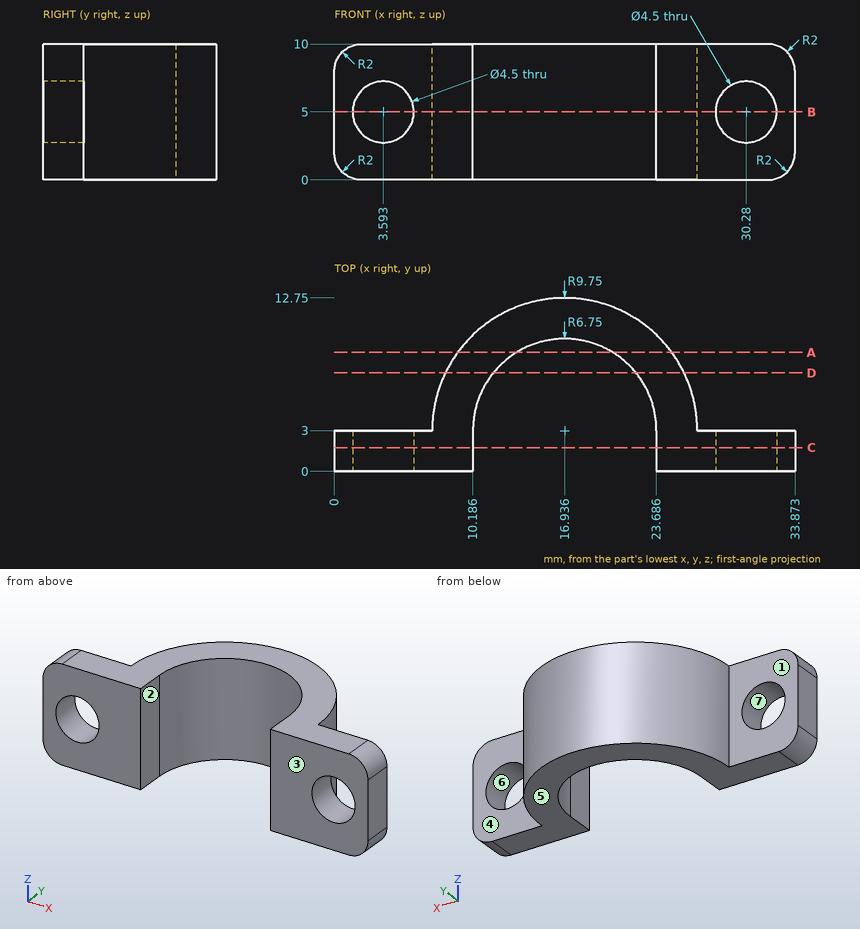
Part print with two shaded views. Sizes in mm from the minimum x, y, z corner. A direction names the side the tool comes from. Give positions to 0.01 mm unless a question says otherwise; leave off trailing zeros. Order: outer loops, then holes, each group sorted by start corner. A loop starts at its lowest first (then second) coordinate and runs counter-clockwise, first axis right, second up.
1) Pin check, flat tips, straight feed: pin 1 (1 mm diameter, centred on x = 22, z = 9, fed in from -Y); pin 2 (3.5 mm diameter, centred on x = 31.5, z = 6, fed in from +Y). Stop position of each tip, or through.
2) Saw through at B-B, the plane z = 5. Write the cut outline in (x, y).
3) Wall check: probe 1 along X at (y, z) = (2.2, 5); probe 2 along Y at (x, z) = (6.5, 9.5); probe 3 along X at (y, z) = (7.75, 6.5). Give the ranges that are in metal, low to high.
4) Saw through at A-A, the plane y = 8.75. Write the cut outline in (x, z).
5) Saw through at D-D, the plane y = 7.25. Write the cut outline in (x, z).
6) Saw through at C-C, the plane y = 1.75. Write the cut outline in (x, z).
7) Mould opens along Z. For the marked faces 4, 5, 6 and 7 say: +Z half, -Z half, draft (parallel to the pull), parting line (faces both ways), or undercut.
8) 3-axis set-ups, long thin cutter, end or side, ignore diameter. For the marked faces 1, 2 and 3: which of +Z, -Z, +X, -X, +Y, -Y reach the whole face in a straight line?
Computed:
1. pin 1: stops at y = 6.82
1. pin 2: stops at y = 3
2. outline: (0, 0) - (1.34, 0) - (1.34, 3) - (0, 3) - close; (5.84, 0) - (10.19, 0) - (10.19, 3) arc R6.75 cw to (23.69, 3) - (23.69, 0) - (28.03, 0) - (28.03, 3) - (26.69, 3) arc R9.75 ccw to (7.19, 3) - (5.84, 3) - close; (32.53, 0) - (33.87, 0) - (33.87, 3) - (32.53, 3) - close
3. probe 1: x = 0 to 1.34, 5.84 to 10.19, 23.69 to 28.03, 32.53 to 33.87
3. probe 2: y = 0 to 3
3. probe 3: x = 8.42 to 12.14, 21.73 to 25.45
4. outline: (9.06, 0) - (13.4, 0) - (13.4, 10) - (9.06, 10) - close; (20.47, 0) - (24.81, 0) - (24.81, 10) - (20.47, 10) - close
5. outline: (8.16, 0) - (11.69, 0) - (11.69, 10) - (8.16, 10) - close; (22.18, 0) - (25.71, 0) - (25.71, 10) - (22.18, 10) - close
6. outline: (0, 2) arc R2 ccw to (2, 0) - (10.19, 0) - (10.19, 10) - (2, 10) arc R2 ccw to (0, 8) - close; (23.69, 0) - (31.87, 0) arc R2 ccw to (33.87, 2) - (33.87, 8) arc R2 ccw to (31.87, 10) - (23.69, 10) - close; hole circle Ø4.5 at (3.59, 5); hole circle Ø4.5 at (30.28, 5)
7. face 4: draft
7. face 5: -Z half
7. face 6: undercut
7. face 7: undercut
8. face 1: +Z, -Z, -X, +Y
8. face 2: +Z, -Z, -Y
8. face 3: +Z, -Z, +X, -X, -Y
